```python
from build123d import *

# Parameters (mm, degrees)
SKETCH_1_R      = 0.9
EXTRUDE_1_DEPTH = 2


with BuildPart() as part:
    # 草图1 → 凸台-拉伸1 (new body)
    with BuildSketch(Plane.XY):
        with BuildLine():
            Line((-29.812520549, 11), (29.812520549, 11))
            ThreePointArc((29.812520549, 11), (31.933840892, 10.121320344), (32.812520549, 8))
            Line((32.812520549, 8), (32.812520549, -8))
            ThreePointArc((32.812520549, -8), (31.933840892, -10.121320344), (29.812520549, -11))
            Line((29.812520549, -11), (-29.812520549, -11))
            ThreePointArc((-29.812520549, -11), (-31.933840892, -10.121320344), (-32.812520549, -8))
            Line((-32.812520549, -8), (-32.812520549, 8))
            ThreePointArc((-32.812520549, 8), (-31.933840892, 10.121320344), (-29.812520549, 11))
        make_face()
        with Locations((2.772967143, 0)):
            Circle(SKETCH_1_R, mode=Mode.SUBTRACT)
        with Locations((30.172967143, 0)):
            Circle(SKETCH_1_R, mode=Mode.SUBTRACT)
        with Locations(Location((-30.172967143, 0, 0), (0, 0, 180))):
            Circle(SKETCH_1_R, mode=Mode.SUBTRACT)
        with Locations(Location((-2.772967143, 0, 0), (0, 0, 180))):
            Circle(SKETCH_1_R, mode=Mode.SUBTRACT)
        with BuildLine():
            Line((4.622967163, 2.40000001), (4.422967163, 2.40000001))
            ThreePointArc((4.422967163, 2.40000001), (4.069413775, 2.253553402), (3.922967167, 1.900000014))
            Line((3.922967167, 1.900000014), (3.922967167, -2.099999986))
            ThreePointArc((3.922967167, -2.099999986), (4.069413775, -2.453553374), (4.422967163, -2.599999982))
            Line((4.422967163, -2.599999982), (4.622967163, -2.599999982))
            ThreePointArc((4.622967163, -2.599999982), (4.976520556, -2.746446592), (5.122967167, -3.099999986))
            Line((5.122967167, -3.099999986), (5.122967167, -6.449999996))
            Line((5.122967167, -6.449999996), (7.622967155, -6.449999996))
            ThreePointArc((7.622967155, -6.449999996), (7.976520542, -6.596446604), (8.12296715, -6.949999991))
            Line((8.12296715, -6.949999991), (8.12296715, -8.45))
            Line((8.12296715, -8.45), (24.822967148, -8.45))
            Line((24.822967148, -8.45), (24.822967148, -6.949999996))
            ThreePointArc((24.822967148, -6.949999996), (24.969413756, -6.596446609), (25.322967143, -6.450000001))
            Line((25.322967143, -6.450000001), (27.822967124, -6.450000001))
            Line((27.822967124, -6.450000001), (27.822967124, 6.250000022))
            Line((27.822967124, 6.250000022), (25.322967143, 6.250000022))
            ThreePointArc((25.322967143, 6.250000022), (24.969413756, 6.39644663), (24.822967148, 6.750000017))
            Line((24.822967148, 6.750000017), (24.822967148, 8.45))
            Line((24.822967148, 8.45), (8.122967152, 8.45))
            Line((8.122967152, 8.45), (8.122967152, 6.949999996))
            ThreePointArc((8.122967152, 6.949999996), (7.976520544, 6.596446609), (7.622967157, 6.450000001))
            Line((7.622967157, 6.450000001), (5.122967167, 6.450000001))
            Line((5.122967167, 6.450000001), (5.122967167, 2.900000014))
            ThreePointArc((5.122967167, 2.900000014), (4.976520556, 2.54644662), (4.622967163, 2.40000001))
        make_face(mode=Mode.SUBTRACT)
        with BuildLine():
            Line((-3.922967167, 1.900000014), (-3.922967167, -2.099999986))
            ThreePointArc((-3.922967167, -2.099999986), (-4.069413775, -2.453553374), (-4.422967163, -2.599999982))
            Line((-4.422967163, -2.599999982), (-4.622967163, -2.599999982))
            ThreePointArc((-4.622967163, -2.599999982), (-4.976520556, -2.746446592), (-5.122967167, -3.099999986))
            Line((-5.122967167, -3.099999986), (-5.122967167, -6.449999996))
            Line((-5.122967167, -6.449999996), (-7.622967155, -6.449999996))
            ThreePointArc((-7.622967155, -6.449999996), (-7.976520542, -6.596446604), (-8.12296715, -6.949999991))
            Line((-8.12296715, -6.949999991), (-8.12296715, -8.45))
            Line((-8.12296715, -8.45), (-24.822967148, -8.45))
            Line((-24.822967148, -8.45), (-24.822967148, -6.949999996))
            ThreePointArc((-24.822967148, -6.949999996), (-24.969413756, -6.596446609), (-25.322967143, -6.450000001))
            Line((-25.322967143, -6.450000001), (-27.822967124, -6.450000001))
            Line((-27.822967124, -6.450000001), (-27.822967124, 6.250000022))
            Line((-27.822967124, 6.250000022), (-25.322967143, 6.250000022))
            ThreePointArc((-25.322967143, 6.250000022), (-24.969413756, 6.39644663), (-24.822967148, 6.750000017))
            Line((-24.822967148, 6.750000017), (-24.822967148, 8.45))
            Line((-24.822967148, 8.45), (-8.122967152, 8.45))
            Line((-8.122967152, 8.45), (-8.122967152, 6.949999996))
            ThreePointArc((-8.122967152, 6.949999996), (-7.976520544, 6.596446609), (-7.622967157, 6.450000001))
            Line((-7.622967157, 6.450000001), (-5.122967167, 6.450000001))
            Line((-5.122967167, 6.450000001), (-5.122967167, 2.900000014))
            ThreePointArc((-5.122967167, 2.900000014), (-4.976520556, 2.54644662), (-4.622967163, 2.40000001))
            Line((-4.622967163, 2.40000001), (-4.422967163, 2.40000001))
            ThreePointArc((-4.422967163, 2.40000001), (-4.069413775, 2.253553402), (-3.922967167, 1.900000014))
        make_face(mode=Mode.SUBTRACT)
    extrude(amount=EXTRUDE_1_DEPTH)


solid = part.part
```
Source: CAD feature listing. Evaluate the final solid. Frame: model axes, mm. A direction names the side the tool comes from. Give positions to 0.01 mm unless a question says otherwise; leave off trailing zeros. Write each loop counter-clockwise with the first axis right and the second up, starting at its lowest first coordinate (ties: lowest second). Pieces come first, ordered by that corner, then holes.
1. Pull-direction query (X, two-part tool) for faces 1 (the face through (0, 0, 0)), 2 (the face through (32.813, 0, 1)), 3 (the face through (-8.123, -8, 1)), 4 (the face through (6, -6.45, 1)); classes: +X half, -X half, draft (parallel to the pull), parting line (faces both ways), or undercut.
2. Material intervals for line 1 along X through (y, z) = (-4.5, 1); line 2 along Y through (x, z) = (11.5, 1.4); line 3 along Y through (x, z) = (6.5, 1.3), sorted ascending.
3. Section query C-C (z = 0.8). Count the separate pieces of the cut face and the enclosed holes in it, then the cut area to 3 significant figures.
4. Section query A-A (y = 0). Return the cut outline in (x, z), then the cut area to 3 significant figures.
5. Section query B-B (x = 21.5). Return the cut outline in (y, z).
6. Access query for faces 5 (the face through (-27, 6.25, 1)), 6 (the face through (0, 0, 2)). Directions: +Z, -Z, +X, -X, +Y, -Y. A direction counts if a zero-diameter tool reaches every point of the face in a straight line with its end or side. Return the directions, or none.
Output values:
1. face 1: draft
1. face 2: +X half
1. face 3: undercut
1. face 4: undercut
2. line 1: x = -32.81 to -27.82, -5.12 to 5.12, 27.82 to 32.81
2. line 2: y = -11 to -8.45, 8.45 to 11
2. line 3: y = -11 to -6.45, 6.45 to 11
3. separate pieces: 1
3. enclosed holes: 6
3. area: 695 mm2
4. outline: (-32.81, 0) - (-31.07, 0) - (-31.07, 2) - (-32.81, 2) - close; (-29.27, 0) - (-27.82, 0) - (-27.82, 2) - (-29.27, 2) - close; (-3.92, 0) - (-3.67, 0) - (-3.67, 2) - (-3.92, 2) - close; (-1.87, 0) - (1.87, 0) - (1.87, 2) - (-1.87, 2) - close; (3.67, 0) - (3.92, 0) - (3.92, 2) - (3.67, 2) - close; (27.82, 0) - (29.27, 0) - (29.27, 2) - (27.82, 2) - close; (31.07, 0) - (32.81, 0) - (32.81, 2) - (31.07, 2) - close
4. area: 21.3 mm2
5. outline: (-11, 0) - (-8.45, 0) - (-8.45, 2) - (-11, 2) - close; (8.45, 0) - (11, 0) - (11, 2) - (8.45, 2) - close
6. face 5: +Z, -Z
6. face 6: +Z, +X, -X, +Y, -Y
